Source: CAD feature listing. Evaluate the final solid. Frame: model axes, mm. A direction names the side the tool comes from. Round coordinates to 2 decimals unless told otherwise and drop trailing zeros. Order: outer loops, then holes, each group sorted by start corner. A loop starts at its lowest first (then second) coordinate and runs counter-clockwise, first axis right, second up. Notation, with made-up numbers: (-3, 46) -> (46, 46) arc R24 cw to (46, 72) -> close; hole circle Ø1 at (42.5, 34.25). An arc over 180 degrees is marked (long way). One line per item, written item: value. Start each with the question number.
1) Ray query, L1, parallel to X at y = 1.25, z = 12.4; L2, parallel to Z at x = 37.4, y = 4.5; L3, parallel to Z at x = -37, y = 3. Return the intervals inside material, ascending.
2) Section D-D (y = 45.5). Return the cut outline in (x, z), and give its area (3 significant figures).
3) Section C-C (x = 37.4). Return the cut outline in (y, z), and give its area (3 significant figures).
4) Pin query (flat end, axial travel): P1, Ø3, axis at y = 2.5, z = -35.5, coming from the +X side; P2, Ø9, axis at x = -7.5, y = 115.5, coming from the -Z side; P3, Ø24, axis at x = -6.5, y = 99, coming from the +Z side. Return the tip coordinate at first contact, or that it passes through.
5) Mould query, pull axis Z, two halves, no side actions, for faces 1 (the face through (-18.2, 3, -30)), 2 (the face through (0, 99, 15)), 3 (the face through (-40, 3, 12.3)). Classes: pulls with the +Z half, pulls with the -Z half, needs draft (parallel to the pull), parting line crosses it, or undercut.
6) Section B-B (z = -12.4). Return the cut outline in (x, y).
7) Reachability of faces 4 (the face through (18.2, 3, 30)), 5 (the face through (15, 3, 37.5)), 6 (the face through (31, 3, -18.2)), 7 (the face through (-31, 3, -18.2)), 8 (the face through (-3, 82, 10)) from +Z, -Z, +X, -X, +Y, -Y: full face, straight path, thin tool, end or side. Return the list, or none.
8) Section A-A (x = -5.5). Return the cut outline in (y, z), and give its area (3 significant figures).
```python
from build123d import *

# Parameters (mm, degrees)
SKETCH_1_W                  = 86
SKETCH_1_H                  = 86
EXTRUDE_1_DEPTH             = 6
SKETCH_2_W                  = 30
SKETCH_2_H                  = 30
EXTRUDE_2_DEPTH             = 160
EXTRUDE_3_REACH             = 173.167
EXTRUDE_3_DIRECTION_2_REACH = 173.167
SKETCH_8_R                  = 2.6
CUT_EXTRUDE_2_DEPTH         = 6
CUT_EXTRUDE_3_DEPTH         = 6
PATTERN_LINEAR_1_COUNT      = 3
PATTERN_LINEAR_1_PITCH      = 45.6
MIRROR_7_COPY_1_DEPTH       = 6
MIRROR_8_COPY_1_SKETCH_R    = 2.6
MIRROR_8_COPY_1_DEPTH       = 6
PATTERN_CIRCULAR_1_COUNT    = 2
PATTERN_CIRCULAR_1_ANGLE    = 90
MIRROR_9_COPY_1_SKETCH_R    = 2.6
MIRROR_9_COPY_1_DEPTH       = 6
MIRROR_9_COPY_2_SKETCH_R    = 2.6
MIRROR_9_COPY_2_DEPTH       = 6
MIRROR_10_COPY_1_SKETCH_R   = 2.6
MIRROR_10_COPY_1_DEPTH      = 6
MIRROR_10_COPY_2_SKETCH_R   = 2.6
MIRROR_10_COPY_2_DEPTH      = 6
MIRROR_10_COPY_3_SKETCH_R   = 2.6
MIRROR_10_COPY_3_DEPTH      = 6
MIRROR_10_COPY_4_SKETCH_R   = 2.6
MIRROR_10_COPY_4_DEPTH      = 6
MIRROR_10_COPY_5_SKETCH_R   = 2.6
MIRROR_10_COPY_5_DEPTH      = 6
EXTRUDE_4_DEPTH             = 15
CUT_EXTRUDE_4_DEPTH         = 9.5
CUT_EXTRUDE_4_DEPTH_BACK    = 172.166585524
SKETCH_17_W                 = 20
SKETCH_17_H                 = 154
SKETCH_19_W                 = 24.8
SKETCH_19_H                 = 5.2
CUT_EXTRUDE_6_DEPTH         = 172.166585524
CUT_EXTRUDE_8_DEPTH         = 9.5
CUT_EXTRUDE_8_DEPTH_BACK    = 172.166585524
SKETCH_21_W                 = 17
SKETCH_21_H                 = 6


with BuildPart() as part:
    # 草图1 → 凸台-拉伸1 (new body)
    with BuildSketch(Plane(origin=(0, 0, 0), x_dir=(1, 0, 0), z_dir=(0, 1, 0))):
        Rectangle(SKETCH_1_W, SKETCH_1_H)
    extrude(amount=EXTRUDE_1_DEPTH)

    # 草图2 → 凸台-拉伸2 (add)
    with BuildSketch(Plane(origin=(0, 0, 0), x_dir=(1, 0, 0), z_dir=(0, 1, 0))):
        Rectangle(SKETCH_2_W, SKETCH_2_H)
    extrude(amount=EXTRUDE_2_DEPTH)

    # 凸台-拉伸3: up to this face of the body (flat: up to its plane)
    extrude_3_end = Plane(part.part.faces().sort_by_distance((0, 83, 15))[0])
    # 草图7 → 凸台-拉伸3 (add, up to the picked face)
    with BuildSketch(Plane.XY, mode=Mode.PRIVATE) as extrude_3_sk1:
        Polygon((-15, 36), (-33, 6), (-15, 6), align=None)
    extrude_3_tool1 = split(extrude(extrude_3_sk1.sketch, amount=EXTRUDE_3_REACH, mode=Mode.PRIVATE), bisect_by=extrude_3_end, keep=Keep.BOTH, mode=Mode.PRIVATE)
    add(extrude_3_tool1.solids().sort_by(Axis((-21, 16, 0), (0, 0, 1)))[0])

    # 凸台-拉伸3 direction 2: up to this face of the body (flat: up to its plane)
    extrude_3_direction_2_end = Plane(part.part.faces().sort_by_distance((0, 83, -15))[0])
    # 草图7 → 凸台-拉伸3 direction 2 (add, up to the picked face)
    with BuildSketch(Plane.XY, mode=Mode.PRIVATE) as extrude_3_direction_2_sk1:
        Polygon((-15, 36), (-33, 6), (-15, 6), align=None)
    extrude_3_direction_2_tool1 = split(extrude(extrude_3_direction_2_sk1.sketch, amount=-EXTRUDE_3_DIRECTION_2_REACH, mode=Mode.PRIVATE), bisect_by=extrude_3_direction_2_end, keep=Keep.BOTH, mode=Mode.PRIVATE)
    add(extrude_3_direction_2_tool1.solids().sort_by(Axis((-21, 16, 0), (0, 0, -1)))[0])

    # 草图8 → 切除-拉伸2 (cut)
    with BuildSketch(Plane(origin=(0, 0, 0), x_dir=(1, 0, 0), z_dir=(0, 1, 0))):
        with Locations(Location((-12.4, 37.4, 0), (0, 0, 270))):
            Circle(SKETCH_8_R)
    cut_extrude_2 = extrude(amount=CUT_EXTRUDE_2_DEPTH, mode=Mode.SUBTRACT)

    # 镜向2: 切除-拉伸2 across plane
    add(cut_extrude_2.mirror(Plane.XY), mode=Mode.SUBTRACT)

    # 草图11 → 切除-拉伸3 (cut)
    with BuildSketch(Plane(origin=(0, 0, 0), x_dir=(1, 0, 0), z_dir=(0, 1, 0))):
        Polygon((264.106039705, -18.2), (43, -18.2), (18.2, -18.2), (18.2, -43), (18.2, -264.106039705), (330.891160074, -576.797199779), (576.797199779, -330.891160074), align=None)
    cut_extrude_3 = extrude(amount=CUT_EXTRUDE_3_DEPTH, mode=Mode.SUBTRACT)

    # 草图12 → 切除-旋转2 (revolve, cut)
    with BuildSketch(Plane.XY):
        with BuildLine():
            Line((15, 62), (15, 42))
            ThreePointArc((15, 42), (5, 52), (15, 62))
        make_face()
    cut_revolve_2 = revolve(axis=Axis((15, 62, 0), (0, -1, 0)), mode=Mode.SUBTRACT)

    # 阵列(线性)1: 切除-旋转2 ×3
    with Locations(*[(0, i * PATTERN_LINEAR_1_PITCH, 0) for i in range(1, PATTERN_LINEAR_1_COUNT)]):
        add(cut_revolve_2, mode=Mode.SUBTRACT)

    # 镜向6: 切除-拉伸3 across plane
    add(cut_extrude_3.mirror(Plane.XY), mode=Mode.SUBTRACT)

    # 镜向7: 切除-拉伸3 across plane
    add(cut_extrude_3.mirror(Plane(origin=(0, 0, 0), x_dir=(0, 0, 1), z_dir=(1, 0, 0))), mode=Mode.SUBTRACT)

    # 镜向7 copy 1 sketch → 镜向7 copy 1 (cut)
    with BuildSketch(Plane(origin=(0, 0, 0), x_dir=(-1, 0, 0), z_dir=(0, 1, 0))):
        Polygon((264.106039705, -18.2), (43, -18.2), (18.2, -18.2), (18.2, -43), (18.2, -264.106039705), (330.891160074, -576.797199779), (576.797199779, -330.891160074), align=None)
    extrude(amount=MIRROR_7_COPY_1_DEPTH, mode=Mode.SUBTRACT)

    # 镜向8: 切除-拉伸2 across plane
    add(cut_extrude_2.mirror(Plane(origin=(0, 0, 0), x_dir=(0, 0, 1), z_dir=(1, 0, 0))), mode=Mode.SUBTRACT)

    # 镜向8 copy 1 sketch → 镜向8 copy 1 (cut)
    with BuildSketch(Plane(origin=(0, 0, 0), x_dir=(-1, 0, 0), z_dir=(0, 1, 0))):
        with Locations(Location((-12.4, 37.4, 0), (0, 0, 270))):
            Circle(MIRROR_8_COPY_1_SKETCH_R)
    extrude(amount=MIRROR_8_COPY_1_DEPTH, mode=Mode.SUBTRACT)

    # 阵列(圆周)1: 切除-拉伸2 ×2 about axis
    pattern_circular_1_axis = Axis((0, 0, 0), (0, 1, 0))
    for i in range(1, PATTERN_CIRCULAR_1_COUNT):
        add(cut_extrude_2.rotate(pattern_circular_1_axis, i * PATTERN_CIRCULAR_1_ANGLE / (PATTERN_CIRCULAR_1_COUNT - 1)), mode=Mode.SUBTRACT)

    # 镜向9 copy 1 sketch → 镜向9 copy 1 (cut)
    with BuildSketch(Plane.ZX):
        with Locations((-12.4, -37.4)):
            Circle(MIRROR_9_COPY_1_SKETCH_R)
    extrude(amount=MIRROR_9_COPY_1_DEPTH, mode=Mode.SUBTRACT)

    # 镜向9 copy 2 sketch → 镜向9 copy 2 (cut)
    with BuildSketch(Plane(origin=(0, 0, 0), x_dir=(1, 0, 0), z_dir=(0, 1, 0))):
        with Locations((-12.4, -37.4)):
            Circle(MIRROR_9_COPY_2_SKETCH_R)
    extrude(amount=MIRROR_9_COPY_2_DEPTH, mode=Mode.SUBTRACT)

    # 镜向10 copy 1 sketch → 镜向10 copy 1 (cut)
    with BuildSketch(Plane(origin=(0, 0, 0), x_dir=(0, 0, -1), z_dir=(0, 1, 0))):
        with Locations((-12.4, -37.4)):
            Circle(MIRROR_10_COPY_1_SKETCH_R)
    extrude(amount=MIRROR_10_COPY_1_DEPTH, mode=Mode.SUBTRACT)

    # 镜向10 copy 2 sketch → 镜向10 copy 2 (cut)
    with BuildSketch(Plane(origin=(0, 0, 0), x_dir=(-1, 0, 0), z_dir=(0, 1, 0))):
        with Locations((-12.4, -37.4)):
            Circle(MIRROR_10_COPY_2_SKETCH_R)
    extrude(amount=MIRROR_10_COPY_2_DEPTH, mode=Mode.SUBTRACT)

    # 镜向10 copy 3 sketch → 镜向10 copy 3 (cut)
    with BuildSketch(Plane.ZX):
        with Locations(Location((-12.4, 37.4, 0), (0, 0, 270))):
            Circle(MIRROR_10_COPY_3_SKETCH_R)
    extrude(amount=MIRROR_10_COPY_3_DEPTH, mode=Mode.SUBTRACT)

    # 镜向10 copy 4 sketch → 镜向10 copy 4 (cut)
    with BuildSketch(Plane(origin=(0, 0, 0), x_dir=(-1, 0, 0), z_dir=(0, 1, 0))):
        with Locations(Location((-12.4, 37.4, 0), (0, 0, 270))):
            Circle(MIRROR_10_COPY_4_SKETCH_R)
    extrude(amount=MIRROR_10_COPY_4_DEPTH, mode=Mode.SUBTRACT)

    # 镜向10 copy 5 sketch → 镜向10 copy 5 (cut)
    with BuildSketch(Plane(origin=(0, 0, 0), x_dir=(-1, 0, 0), z_dir=(0, 1, 0))):
        with Locations((-12.4, -37.4)):
            Circle(MIRROR_10_COPY_5_SKETCH_R)
    extrude(amount=MIRROR_10_COPY_5_DEPTH, mode=Mode.SUBTRACT)

    # 草图15 → 凸台-拉伸4 (add, symmetric)
    with BuildSketch(Plane(origin=(0, 0, 0), x_dir=(0, 0, -1), z_dir=(1, 0, 0))):
        Polygon((-15, 36), (-15, 6), (-33, 6), align=None)
    extrude_4 = extrude(amount=EXTRUDE_4_DEPTH, both=True)

    # 镜向11: 凸台-拉伸4 across plane
    add(extrude_4.mirror(Plane.XY))

    # 草图17 → 切除-拉伸4 (cut, two sides: drawn at the far end of the back side and taken through both)
    with BuildSketch(Plane(origin=(0, 0, 0), x_dir=(0, 0, -1), z_dir=(1, 0, 0)).offset(-CUT_EXTRUDE_4_DEPTH_BACK)):
        with Locations((0, 83)):
            Rectangle(SKETCH_17_W, SKETCH_17_H)
    extrude(amount=CUT_EXTRUDE_4_DEPTH + CUT_EXTRUDE_4_DEPTH_BACK, mode=Mode.SUBTRACT)

    # 草图19 → 切除-拉伸6 (cut, through all)
    with BuildSketch(Plane(origin=(0, 0, 0), x_dir=(1, 0, 0), z_dir=(0, 1, 0))):
        with Locations((0, 37.4)):
            Rectangle(SKETCH_19_W, SKETCH_19_H)
    cut_extrude_6 = extrude(amount=CUT_EXTRUDE_6_DEPTH, mode=Mode.SUBTRACT)

    # 镜向12: 切除-拉伸6 across plane
    add(cut_extrude_6.mirror(Plane.XY), mode=Mode.SUBTRACT)

    # 草图21 → 切除-拉伸8 (cut, two sides: drawn at the far end of the back side and taken through both)
    with BuildSketch(Plane(origin=(0, 0, 0), x_dir=(0, 0, -1), z_dir=(1, 0, 0)).offset(-CUT_EXTRUDE_8_DEPTH_BACK)):
        with Locations((0, 3)):
            Rectangle(SKETCH_21_W, SKETCH_21_H)
    extrude(amount=CUT_EXTRUDE_8_DEPTH + CUT_EXTRUDE_8_DEPTH_BACK, mode=Mode.SUBTRACT)


solid = part.part
```
Findings:
1. L1: -43 to -40, -34.8 to 34.8, 40 to 43
1. L2: -18.2 to -15, -9.8 to 9.8, 15 to 18.2
1. L3: -18.2 to -14.97, -9.83 to -8.5, 8.5 to 9.83, 14.97 to 18.2
2. outline: (-15, -15) -> (15, -15) -> (15, -7.6) arc R7.6 cw to (9.5, -5.24) -> (9.5, -10) -> (-15, -10) -> close; (-15, 10) -> (9.5, 10) -> (9.5, 5.24) arc R7.6 cw to (15, 7.6) -> (15, 15) -> (-15, 15) -> close
2. area: 334 mm2
3. outline: (0, -18.2) -> (6, -18.2) -> (6, -15) -> (0, -15) -> close; (0, -9.8) -> (6, -9.8) -> (6, 9.8) -> (0, 9.8) -> close; (0, 15) -> (6, 15) -> (6, 18.2) -> (0, 18.2) -> close
3. area: 156 mm2
4. P1: x = 18.2
4. P2: z = -15
4. P3: z = 15
5. face 1: needs draft
5. face 2: pulls with the +Z half
5. face 3: undercut
6. outline: (-43, 0) -> (-40, 0) -> (-40, 6) -> (-43, 6) -> close; (-34.8, 0) -> (34.8, 0) -> (34.8, 6) -> (15, 6) -> (15, 160) -> (-15, 160) -> (-15, 36) -> (-33, 6) -> (-34.8, 6) -> close; (40, 0) -> (43, 0) -> (43, 6) -> (40, 6) -> close
7. face 4: +Z, +X, +Y, -Y
7. face 5: +Y, -Y
7. face 6: -Z, +X, +Y, -Y
7. face 7: -Z, -X, +Y, -Y
7. face 8: -X, +Y
8. outline: (0, -43) -> (6, -43) -> (6, -40) -> (0, -40) -> close; (0, -34.8) -> (6, -34.8) -> (6, -33) -> (36, -15) -> (160, -15) -> (160, -10) -> (6, -10) -> (6, -8.5) -> (0, -8.5) -> close; (0, 8.5) -> (6, 8.5) -> (6, 10) -> (160, 10) -> (160, 15) -> (36, 15) -> (6, 33) -> (6, 34.8) -> (0, 34.8) -> close; (0, 40) -> (6, 40) -> (6, 43) -> (0, 43) -> close
8. area: 2,430 mm2
